Autodesk Inventor part; units mm, degrees
ref_plane "YZ Plane" through (0, 0, 0) normal (1, 0, 0) x (0, 1, 0)
ref_plane "XZ Plane" through (0, 0, 0) normal (0, 1, 0) x (-1, 0, 0)
ref_plane "XY Plane" through (0, 0, 0) normal (0, 0, 1) x (1, 0, 0)
sketch "Sketch1" plane through (0, 0, 0) normal (0, 1, 0) x (-1, 0, 0)
  line L0 (-17.75, 62.5) -> (17.75, 62.5)
  line L1 (17.75, 62.5) -> (17.75, -62.5)
  line L2 (17.75, -62.5) -> (-17.75, -62.5)
  line L3 (-17.75, -62.5) -> (-17.75, 62.5)
  line L4 (-17.75, 62.5) -> (17.75, -62.5) construction
  line L5 (17.75, 62.5) -> (-17.75, -62.5) construction
  point P0 (0, 0)
  dimension "d0" = 35.5
  dimension "d1" = 125
extrude "Extrusion1" add sketch "Sketch1" along normal blind 1.6
sketch "Sketch2" plane through (0, 1.6, 0) normal (0, 1, 0) x (1, 0, 0)
  line L0 (17.75, 62.5) -> (-17.75, 62.5)
  line L1 (-17.75, -62.5) -> (17.75, -62.5)
  line L2 (-17.75, 62.5) -> (-16.15, 62.5)
  line L3 (-16.15, 62.5) -> (-16.15, -62.5)
  line L4 (-16.15, -62.5) -> (-17.75, -62.5)
  line L5 (-17.75, -62.5) -> (-17.75, 62.5)
  point P0 (0, 0)
  dimension "d4" = 1.6
extrude "Extrusion2" add sketch "Sketch2" along normal blind 17.6
sketch "Sketch3" plane through (-17.75, 0, -62.5) normal (-1, 0, 0) x (0, 0, 1)
  line L0 (62.5, 0) -> (62.5, 72.1121) construction
  line L1 (98.5, 0) -> (26.5, 0) construction
  line L2 (26.5, 0) -> (26.5, 19.2) construction
  line L3 (26.5, 19.2) -> (98.5, 19.2) construction
  line L4 (98.5, 19.2) -> (98.5, 0) construction
  line L5 (98.5, 0) -> (26.5, 19.2) construction
  line L6 (26.5, 0) -> (98.5, 19.2) construction
  line L7 (0, 19.2) -> (125, 19.2) construction
  line L8 (125, 0) -> (0, 0) construction
  line L9 (125, 19.2) -> (87, 19.2)
  line L10 (87, 19.2) -> (87, 6)
  line L11 (87, 6) -> (125, 6)
  line L12 (125, 6) -> (125, 19.2)
  line L13 (0, 19.2) -> (38, 19.2)
  line L14 (38, 19.2) -> (38, 6)
  line L15 (38, 6) -> (0, 6)
  line L16 (0, 6) -> (0, 19.2)
  point P0 (62.5, 9.6)
  dimension "d7" = 72
  dimension "d8" = 38
  dimension "d9" = 6
extrude "Extrusion3" cut sketch "Sketch3" against normal through all
sketch "Sketch4" plane through (-17.75, 0, -62.5) normal (-1, 0, 0) x (0, 0, 1)
  line L0 (62.5, 0) -> (62.5, 59.5527) construction
  line L1 (44.75, 6) -> (80.25, 6) construction
  line L2 (80.25, 6) -> (80.25, 0) construction
  line L3 (80.25, 0) -> (44.75, 0) construction
  line L4 (44.75, 0) -> (44.75, 6) construction
  line L5 (44.75, 6) -> (80.25, 0) construction
  line L6 (80.25, 6) -> (44.75, 0) construction
  line L7 (125, 0) -> (0, 0) construction
  point P0 (62.5, 3)
  dimension "d12" = 6
  dimension "d13" = 35.5
hole "Hole1" at (-17.75, 6, 17.75) at (-17.75, 6, -17.75) direction (1, 0, 0) diameter 3 end through all
properties part number "fitplate"
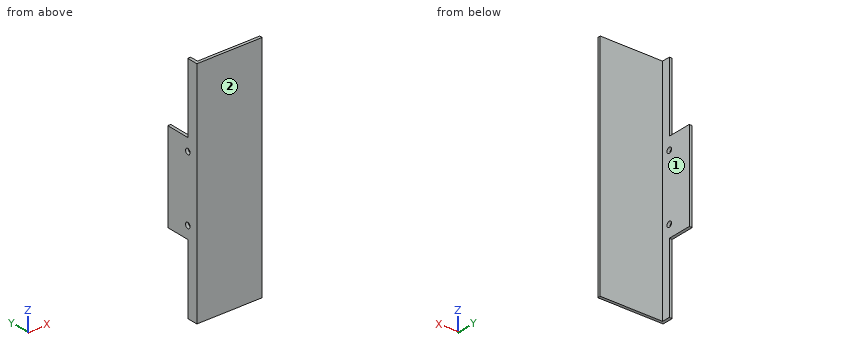
Verification items for the finished model (mm, model axes). Face numbers are marked on the shaded views. A direction names the side the tool comes from. Give positions to 0.01 mm unless a question says otherwise; leave off trailing zeros. Order: outer loops, then holes, each group sorted by start corner. A loop starts at its lowest first (then second) coordinate and runs counter-clockwise, first axis right, second up. Notation, with made-up numbers: M -31.5,29 L -1.5,29 A24 cw -1.5,47 Z; hole C 71,12.5 d8. An arc over 180 degrees is marked long. Answer in a Markdown table with one row per item. Add a question column.
Item 1: Section check B-B, the plane x = -5.5. Enter the section's corners in (y, z).
Item 2: Section check A-A, the plane z = 17.75. Enter the section's corners in (x, y).
Item 3: Gauge pin test, flat ends, axial feed: pin 1 (1.8 mm diameter, centred on x = -17, z = 45.5, fed in from +Y); pin 2 (6 mm diameter, centred on x = 0.5, y = 5, fed in from +Z); pin 3 (3 mm diameter, centred on x = 9, z = 26, fed in from +Y); pin 4 (1.8 mm diameter, centred on x = -17.5, y = 15.5, fed in from -Z). Record the tip position at first contact, or that the pin passes through.
Item 4: Section check C-C, the plane z = -45.5. Enter the section's corners in (x, y).
Item 5: Tool access check on the marked faces 1 and 2. Record the directions out of +Z, -Z, +X, -X, +Y, -Y that give a thin tool (end or side, any length) a straight path to the whole face; none if there is none.
Item 6: Section check D-D, the plane y = 12. Enter the section's corners in (x, z).
Item 7: Scan lines: probe 1 along Y at (x, z) = (-17, -17.75); probe 2 along X at (y, z) = (6.25, -4); probe 3 along Y at (x, z) = (12.5, 49.5). Record each from-to range of solid material in increasing order. Write a range as from..to.
Filled sheet:
| question | item | result |
|---|---|---|
| 1 | outline | M 0,-62.5 L 1.6,-62.5 L 1.6,62.5 L 0,62.5 Z |
| 2 | outline | M -17.75,0 L 17.75,0 L 17.75,1.6 L -16.15,1.6 L -16.15,4.5 L -17.75,4.5 Z; M -17.75,7.5 L -16.15,7.5 L -16.15,19.2 L -17.75,19.2 Z |
| 3 | pin 1 | stops at y = 6 |
| 3 | pin 2 | passes through |
| 3 | pin 3 | stops at y = 1.6 |
| 3 | pin 4 | stops at z = -24.5 |
| 4 | outline | M -17.75,0 L 17.75,0 L 17.75,1.6 L -16.15,1.6 L -16.15,6 L -17.75,6 Z |
| 5 | face 1 | +Z, -Z, +X, +Y |
| 5 | face 2 | +Z, -Z, +X, -X, -Y |
| 6 | outline | M -17.75,-24.5 L -16.15,-24.5 L -16.15,24.5 L -17.75,24.5 Z |
| 7 | probe 1 | y = 0..4.5, 7.5..19.2 |
| 7 | probe 2 | x = -17.75..-16.15 |
| 7 | probe 3 | y = 0..1.6 |
